from build123d import *

# Parameters (mm, degrees)
SKETCH1_W           = 35
SKETCH1_H           = 8
SKETCH1_R           = 1.35
BOSS_EXTRUDE1_DEPTH = 2
SKETCH2_W           = 35
SKETCH2_H           = 2
BOSS_EXTRUDE3_DEPTH = 30


with BuildPart() as part:
    # Sketch1 → Boss-Extrude1 (new body)
    with BuildSketch(Plane.XY):
        Rectangle(SKETCH1_W, SKETCH1_H)
        with Locations((12, 0)):
            Circle(SKETCH1_R, mode=Mode.SUBTRACT)
        with Locations(Location((-12, 0, 0), (0, 0, 180))):
            Circle(SKETCH1_R, mode=Mode.SUBTRACT)
    extrude(amount=BOSS_EXTRUDE1_DEPTH)

    # Sketch2 → Boss-Extrude3 (add)
    with BuildSketch(Plane.XY.offset(2)):
        with Locations((0, 3)):
            Rectangle(SKETCH2_W, SKETCH2_H)
    extrude(amount=BOSS_EXTRUDE3_DEPTH)


solid = part.part
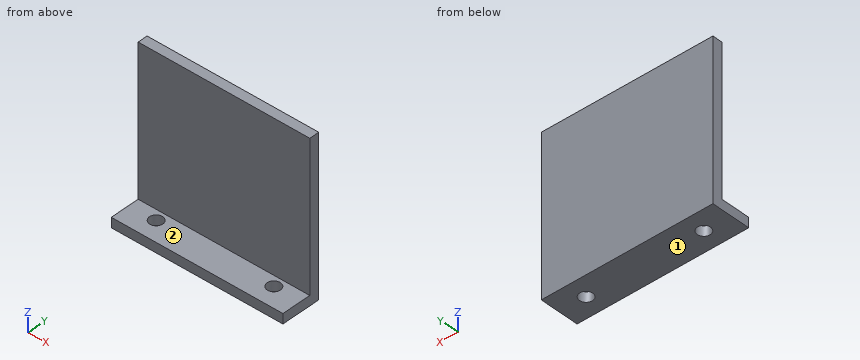
Can you work these out from the model? Positions are in its coordinate system, mm. Face numbers are marked on the shaded views. A direction names the side the tool comes from. Round coordinates to 2 decimals unless told otherwise and drop trailing zeros. Order: outer loops, then holes, each group sorted by start corner. A loop starts at its lowest first (then second) coordinate and runs counter-clockwise, first axis right, second up. Notation, with made-up numbers: M 85,76.25 L 89,76.25 A29 cw 89,96.25 Z; hole C 32,47.5 d4. An arc over 180 degrees is marked long. Use a Markdown table: item, result.
1) On a 3-axis mill with a long thin cutter (end or side, diameter ignored), from which of +Z, -Z, +X, -X, +Y, -Y can I reach the whole of each face in a straight line? I mean the marked faces 1 and 2. Say none if no direction works.
Geometry says:
| item | result |
|---|---|
| face 1 | -Z, +X, -X, +Y, -Y |
| face 2 | +Z, +X, -X, -Y |
2) Imagine slicing it at A-A (x = -12). List the corners of the cut face in (y, z) for me, then the cut area to 3 significant figures.
Geometry says:
| item | result |
|---|---|
| outline | M -4,0 L -1.35,0 L -1.35,2 L -4,2 Z; M 1.35,0 L 4,0 L 4,32 L 2,32 L 2,2 L 1.35,2 Z |
| area | 70.6 mm² |
3) I'm going to push flat-ended pins straight in: P1, Ø15, axis at x = -0.5, z = 11, coming from the -Y side; P2, Ø3, axis at x = 7.5, y = -2, coming from the +Z side; P3, Ø2.5, axis at x = 12, y = 0, coming from the -Z side. Where does each tip first touch, or does it pass through?
Geometry says:
| item | result |
|---|---|
| P1 | stops at y = 2 |
| P2 | stops at z = 2 |
| P3 | passes through |
4) If I drill on line 1 along Y through (x, z) = (12, 1); line 2 along Y through (x, z) = (10, 21); line 3 along Z through (x, y) = (-2, 1), over which ranges is the centre line in solid material (lowest first)?
Geometry says:
| item | result |
|---|---|
| line 1 | y = -4 to -1.35, 1.35 to 4 |
| line 2 | y = 2 to 4 |
| line 3 | z = 0 to 2 |
5) Imagine slicing it at B-B (y = 0). List the corners of the cut face in (x, z) for me.
Geometry says:
| item | result |
|---|---|
| outline | M -17.5,0 L -13.35,0 L -13.35,2 L -17.5,2 Z; M -10.65,0 L 10.65,0 L 10.65,2 L -10.65,2 Z; M 13.35,0 L 17.5,0 L 17.5,2 L 13.35,2 Z |
6) Imagine slicing it at C-C (x = 7.5). List the corners of the cut face in (y, z) for me, then the cut area to 3 significant figures.
Geometry says:
| item | result |
|---|---|
| outline | M -4,0 L 4,0 L 4,32 L 2,32 L 2,2 L -4,2 Z |
| area | 76.0 mm² |
7) Imagine slicing it at D-D (z = 13.5). List the corners of the cut face in (x, y) for me.
Geometry says:
| item | result |
|---|---|
| outline | M -17.5,2 L 17.5,2 L 17.5,4 L -17.5,4 Z |
